Autodesk Inventor part; units mm, degrees
ref_plane "YZ Plane" through (0, 0, 0) normal (1, 0, 0) x (0, 1, 0)
ref_plane "XZ Plane" through (0, 0, 0) normal (0, 1, 0) x (-1, 0, 0)
ref_plane "XY Plane" through (0, 0, 0) normal (0, 0, 1) x (1, 0, 0)
sketch "Sketch1" plane through (0, 0, 0) normal (0, 1, 0) x (-1, 0, 0)
  circle A0 centre (0, 0) radius 37.5
  line L0 (0, 0) -> (37.5, 0)
  line L1 (37.5, 0) -> (-18.75, 32.476)
  line L2 (37.5, 0) -> (102.4519, 0) construction
  line L3 (-18.75, 32.476) -> (-18.75, -32.476)
  line L4 (37.5, 0) -> (-18.75, -32.476)
  line L5 (37.5, 0) -> (37.5, 160)
  line L6 (37.5, 160) -> (37.5, 180)
  circle A1 centre (37.5, 180) radius 2.25
  circle A2 centre (37.5, 200) radius 2.25
  circle A3 centre (57.5, 180) radius 2.25
  circle A4 centre (57.5, 200) radius 2.25
  line L7 (57.5, 180) -> (67.5, 180)
  line L8 (67.5, 180) -> (67.5, 170)
  line L9 (67.5, 170) -> (7.5, 170)
  line L10 (7.5, 170) -> (7.5, 210)
  line L11 (7.5, 210) -> (67.5, 210)
  line L12 (67.5, 210) -> (67.5, 170)
  line L13 (143.4743, -91.4952) -> (178.1153, -111.4952)
  line L14 (178.1153, -111.4952) -> (148.1153, -163.4567)
  circle A5 centre (154.4551, -132.476) radius 2.25
  circle A6 centre (144.4551, -149.7965) radius 2.25
  line L15 (148.1153, -163.4567) -> (113.4743, -143.4567)
  line L16 (113.4743, -143.4567) -> (143.4743, -91.4952)
  circle A7 centre (127.1346, -139.7965) radius 2.25
  circle A8 centre (137.1346, -122.476) radius 2.25
  circle A9 centre (0, 0) radius 37.5
  line L17 (-150.9743, -78.5048) -> (-185.6153, -98.5048)
  line L18 (-185.6153, -98.5048) -> (-215.6153, -46.5433)
  circle A10 centre (-191.9551, -67.524) radius 2.25
  circle A11 centre (-201.9551, -50.2035) radius 2.25
  line L19 (-215.6153, -46.5433) -> (-180.9743, -26.5433)
  line L20 (-180.9743, -26.5433) -> (-150.9743, -78.5048)
  circle A12 centre (-184.6346, -40.2035) radius 2.25
  circle A13 centre (-174.6346, -57.524) radius 2.25
  circle A14 centre (0, 0) radius 37.5
  circle A15 centre (0, 0) radius 48
  line L21 (-215.6153, -46.5433) -> (-155.6153, -46.5433) construction
  line L22 (67.5, 210) -> (127.5, 210) construction
  line L23 (67.5, 210) -> (15, 210) construction
  line L24 (-215.6153, -46.5433) -> (-185.6153, -46.5433) construction
  line L25 (67.5, 210) -> (22.5, 210) construction
  line L26 (-215.6153, -46.5433) -> (-170.6153, -46.5433) construction
  line L27 (-215.6153, -46.5433) -> (-170.6153, -46.5433) construction
  line L28 (-18.75, -32.476) -> (-41.25, -71.4471)
  line L29 (-18.75, -32.476) -> (26.25, -32.476) construction
  line L30 (-41.25, -71.4471) -> (-84.5513, -46.4471)
  line L31 (-41.25, -71.4471) -> (2.0513, -96.4471)
  line L32 (-41.25, -71.4471) -> (8.75, -71.4471) construction
  line L33 (82.5, 0) -> (82.5, -50)
  line L34 (82.5, 0) -> (82.5, 50)
  line L35 (-41.25, 71.4471) -> (2.0513, 96.4471)
  line L36 (-41.25, 71.4471) -> (-84.5513, 46.4471)
  line L37 (-84.5513, -46.4471) -> (-84.5513, 46.4471)
  line L38 (82.5, -50) -> (2.0513, -96.4471)
  line L39 (82.5, 50) -> (2.0513, 96.4471)
  line L40 (2.0513, -240.7847) -> (-103.75, -179.7003)
  line L41 (-103.75, -179.7003) -> (-209.5513, -118.6159)
  line L42 (-209.5513, -118.6159) -> (-209.5513, 118.6159)
  line L43 (-209.5513, 118.6159) -> (-103.75, 179.7003)
  line L44 (-103.75, 179.7003) -> (2.0513, 240.7847)
  line L45 (2.0513, 240.7847) -> (207.5, 122.1688)
  line L46 (207.5, 122.1688) -> (207.5, 0)
  line L47 (207.5, 0) -> (207.5, -122.1688)
  line L48 (207.5, -122.1688) -> (2.0513, -240.7847)
  point P0 (37.5, 0)
  point P1 (-18.75, 32.476)
  point P2 (37.5, 0)
  dimension "d0" = 75
  dimension "d1" = 37.5
  dimension "d2" = 150
  dimension "d3" = 160
  dimension "d4" = 20
  dimension "d5" = 4.5
  dimension "d8" = 20
  dimension "d11" = 20
  dimension "d14" = 10
  dimension "d15" = 10
  dimension "d16" = 60
  dimension "d17" = 40
  dimension "d20" = 360
  dimension "d22" = 96
  dimension "d45" = 45
  dimension "d46" = 120
  dimension "d47" = 50
  dimension "d48" = 90
  dimension "d49" = 50
  dimension "d50" = 30
  dimension "d53" = 360
  dimension "d72" = 125
ref_plane "Work Plane2" through (0, 3, 0) normal (0, 1, 0) x (1, 0, 0)
ref_plane "Work Plane1" through (0, 3, 0) normal (0, 1, 0) x (1, 0, 0)
extrude "Extrusion8" add sketch "Sketch1" along normal blind 3 contours L1 A0 | L5 A15 L28 A0 | L4 L3 L1 | A0 L4 | A0 L28 A15 L5 | L3 A0 | A15 L28 L30 L37 L36 L35 L39 L5 | L5 L39 L34 L33 L38 L31 L28 A15 | L9 L8 L12 L45 L46 L47 L48 L14 L13 L16 L15 L40 L41 L42 L18 L17 L20 L19 L43 L44 L11 L10 | A1 | A3 | L9 L10 L11 L45 L12 L8 | L48 L15 L16 L13 L14 | L19 L20 L17 L18 L42 | A2 | A4 | A5 | A6 | A7 | A8 | A10 | A11 | A12 | A13
sketch "Sketch4" plane through (0, 3, 0) normal (0, 1, 0) x (1, 0, 0)
  line L0 (0, 0) -> (-150, 0)
  circle A0 centre (0, 0) radius 2.5
  line L1 (-150, 0) -> (-150, -19.995)
  circle A1 centre (-150, -19.995) radius 2.5
  line L2 (-150, 0) -> (-150, 19.995)
  circle A2 centre (-150, 19.995) radius 2.5
  circle A3 centre (-150, 0) radius 2.5
  dimension "d79" = 150
  dimension "d80" = 5
  dimension "d81" = 19.995
  dimension "d82" = 5
  dimension "d83" = 19.995
  dimension "d84" = 5
  dimension "d90" = 5
extrude "Extrusion10" cut sketch "Sketch4" against normal blind 3
pattern_circular "Circular Pattern2" count 3 over 360 about axis through (0, 3, 0) along (0, -1, 0) of "Extrusion10"
sketch "Sketch5" plane through (0, 3, 0) normal (0, 1, 0) x (1, 0, 0)
  circle A0 centre (0, 0) radius 100
  circle A1 centre (0, 0) radius 2.5
  line L0 (0, 0) -> (100, 0)
  line L1 (100, 0) -> (100, 20)
  line L2 (0, 0) -> (50, 86.6025)
  line L3 (0, 0) -> (100, 0) construction
  line L4 (50, 86.6025) -> (67.3205, 76.6025)
  dimension "d96" = 200
  dimension "d97" = 20
  dimension "d98" = 60
  dimension "d99" = 20
properties part number "Delta_Top" material "Glass"
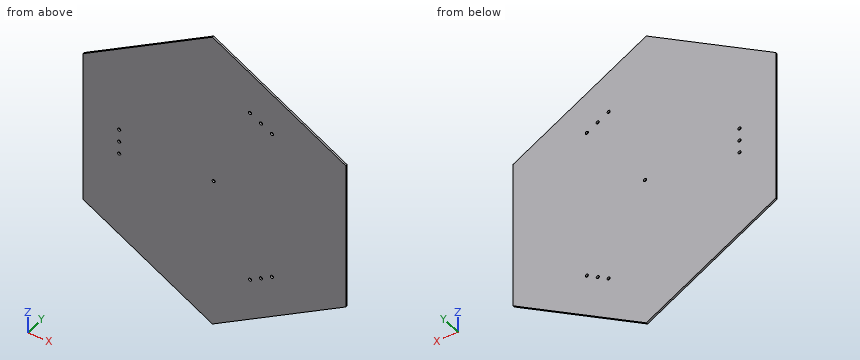
Input: part model. Units: mm. Frame: model coordinates. Coordinates: 2 decimals unless noted, no trailing zeros. Order: outer loops, then holes, each group sorted by start corner. A loop starts at its lowest first (then second) coordinate and runs counter-clockwise, first axis right, second up. Notation, with made-up numbers: M 67.5,-17.5 L 107.5,-17.5 A8 ccw 107.5,-5.5 Z; hole C -20,57 d7. An arc over 180 degrees is marked long. Answer in a Markdown table with one row per item.
(1) Material intervals for line 1 (X direction, y = 2.4, z = 0); line 2 (Z direction, x = 75, y = 2.7); line 3 (Z direction, x = 0, y = 2.35), sorted ascending. Write a range as [from, to].
Numbers:
| item | result |
|---|---|
| line 1 | x = [-207.5, -152.5], [-147.5, -2.5], [2.5, 209.55] |
| line 2 | z = [-196.3, -132.4], [-127.4, 127.4], [132.4, 196.3] |
| line 3 | z = [-239.6, -2.5], [2.5, 239.6] |
(2) Section query B-B, the plane x = -95. Output: boundary loops of the cut face in (y, z).
Numbers:
| item | result |
|---|---|
| outline | M 0,-187.12 L 3,-187.12 L 3,187.12 L 0,187.12 Z |
(3) Section query A-A, the plane y = 2.5. Give the number of separate pieces and of enclosed holes in the cut face, plus the area to 3 significant figures.
Numbers:
| item | result |
|---|---|
| separate pieces | 1 |
| enclosed holes | 10 |
| area | 150,000 mm^2 |
(4) Contact query for flat-ended pins moving along their axis: pin 1 Ø1.5 at (x, y) = (18.5, 2.5) entering from -Z; pin 2 Ø1 at (x, y) = (102.5, 1.5) entering from -Z. Output: stop coordinate, or through.
Numbers:
| item | result |
|---|---|
| pin 1 | stops at z = -229.35 |
| pin 2 | stops at z = -180.71 |
(5) Section query C-C, the plane z = 202. Output: boundary loops of the cut face in (x, y).
Numbers:
| item | result |
|---|---|
| outline | M -69.23,0 L 65.13,0 L 65.13,3 L -69.23,3 Z |
